Part model, mm, in its own coordinate system. Face numbers are marked on the shaded views. A direction names the side the tool comes from. Round coordinates to 2 decimals unless told otherwise and drop trailing zeros. Loops run counter-clockwise (first coordinate to the right, second up) from the corner with the lowest first, then second, coordinate; pieces in that order, holes last. Notation, with made-up numbers: (80.25, -38.75) -> (118.25, -38.75) arc R16 cw to (118.25, -11.75) -> close; hole circle Ø3 at (49.25, 76.5). An arc over 180 degrees is marked (long way). Use a Markdown table: item, result. Add a question column.
Item 1: Which spindle directions (+Z, -Z, +X, -X, +Y, -Y) get a long thin tool onto all of the face, cutting with end or side? Do the marked faces 4, 5, 6 and 7. Say none if no direction does.
Item 2: Cut at D-D, the plane x = 29. List the corners of the cut face in (y, z), plus the area to 3 significant figures.
Item 3: Flat gauge pins, fed straight in: pin 1 (8 mm diameter, centred on x = -211.5, z = -63, fed in from +Y); pin 2 (4 mm diameter, centred on y = 226, z = -13, fed in from -X); pin 3 (12 mm diameter, centred on x = -229.5, y = 222, fed in from +Z). Where does each tip first touch, or does it go through?
Item 4: Cut at B-B, the plane y = 34.5. List the corners of the cut face in (x, z), plus the area to 3 significant figures.
Item 5: Probe line 1 (X direction, y = 229, z = -59); line 2 (X direction, y = 29, z = -60); line 3 (Z direction, x = 96, y = 67). List the from-to ranges inside material, lowest first. Write a range as [from, to].
Item 6: Cut at A-A, the plane x = -135. List the corners of the cut face in (y, z).
Item 7: Cut at C-C, the plane z = 90. List the corners of the cut face in (x, y).
Item 8: Two-plate mould, pull along X, no slides. Class the marked faces 1, 2 and 3: pulls with the +X half, pulls with the -X half, needs draft (parallel to the pull), parting line crosses it, or undercut.
```python
from build123d import *

# Parameters (mm, degrees)
SKETCH1_W                = 400
SKETCH1_H                = 300
BOSS_EXTRUDE1_DEPTH      = 85
SKETCH2_R                = 65
BOSS_EXTRUDE2_DEPTH      = 200
FILLET1_R                = 30
CUT_EXTRUDE1_DEPTH       = 30
RIB1_REACH               = 408.602
SKETCH4_WALL_W           = 996.380250876
SKETCH4_WALL_H           = 30
SKETCH6_R                = 30
CUT_EXTRUDE2_DEPTH       = 380.110801745
SKETCH7_R                = 45
CUT_EXTRUDE3_DEPTH       = 40
CUT_EXTRUDE4_START       = -40
SKETCH8_R                = 45
CUT_EXTRUDE4_DEPTH       = 40
CHAMFER1_SIZE            = 2
BOSS_EXTRUDE3_REACH      = 547.275
BOSS_EXTRUDE3_END_RADIUS = 65
SKETCH9_W                = 16
SKETCH9_H                = 40
FILLET2_R                = 20
CUT_EXTRUDE5_DEPTH       = 424.826615493
CUT_EXTRUDE5_DEPTH_BACK  = 424.826615493
SKETCH10_R               = 10


with BuildPart() as part:
    # Sketch1 → Boss-Extrude1 (new body)
    with BuildSketch(Plane(origin=(0, 0, 0), x_dir=(1, 0, 0), z_dir=(0, 1, 0))):
        Rectangle(SKETCH1_W, SKETCH1_H)
    extrude(amount=BOSS_EXTRUDE1_DEPTH)

    # Sketch2 → Boss-Extrude2 (add)
    with BuildSketch(Plane(origin=(0, 85, 0), x_dir=(1, 0, 0), z_dir=(0, 1, 0))):
        with Locations(Location((-135, 60, 0), (0, 0, 180))):
            Circle(SKETCH2_R)
    extrude(amount=BOSS_EXTRUDE2_DEPTH)

    # Fillet1
    fillet1_edges = [part.edges().sort_by_distance(p)[0] for p in [
        (200, 42.5, 150),
        (-200, 42.5, 150),
        (-200, 42.5, -150),
        (200, 42.5, -150),
    ]]
    fillet(fillet1_edges, radius=FILLET1_R)

    # Sketch3 → Cut-Extrude1 (cut)
    with BuildSketch(Plane(origin=(0, 85, 0), x_dir=(1, 0, 0), z_dir=(0, 1, 0))):
        with BuildLine():
            Line((70, -70), (170, -70))
            ThreePointArc((170, -70), (190, -90), (170, -110))
            Line((170, -110), (70, -110))
            ThreePointArc((70, -110), (50, -90), (70, -70))
        make_face()
    extrude(amount=-CUT_EXTRUDE1_DEPTH, mode=Mode.SUBTRACT)

    # Sketch4 wall → Rib1 (add, up to next)
    with BuildSketch(Plane(origin=(-27.5, 165, -60), x_dir=(-0.469155225962, 0.883115719457, 0), z_dir=(-0.883115719457, -0.469155225962, 0)), mode=Mode.PRIVATE) as rib1_sk1:
        Rectangle(SKETCH4_WALL_W, SKETCH4_WALL_H)
    rib1_tool1 = extrude(rib1_sk1.sketch, amount=RIB1_REACH, mode=Mode.PRIVATE) - part.part
    add(rib1_tool1.solids().sort_by_distance((-27.5, 165, -60))[0])

    # Sketch6 → Cut-Extrude2 (cut, through all)
    with BuildSketch(Plane(origin=(0, 285, 0), x_dir=(1, 0, 0), z_dir=(0, 1, 0))):
        with Locations(Location((-135, 60, 0), (0, 0, 270))):
            Circle(SKETCH6_R)
    extrude(amount=-CUT_EXTRUDE2_DEPTH, mode=Mode.SUBTRACT)

    # Sketch7 → Cut-Extrude3 (cut)
    with BuildSketch(Plane(origin=(0, 0, 0), x_dir=(1, 0, 0), z_dir=(0, 1, 0))):
        with Locations(Location((-135, 60, 0), (0, 0, 270))):
            Circle(SKETCH7_R)
    extrude(amount=CUT_EXTRUDE3_DEPTH, mode=Mode.SUBTRACT)

    # Sketch8 → Cut-Extrude4 (cut)
    with BuildSketch(Plane(origin=(0, 285, 0), x_dir=(1, 0, 0), z_dir=(0, 1, 0)).offset(CUT_EXTRUDE4_START)):
        with Locations(Location((-135, 60, 0), (0, 0, 270))):
            Circle(SKETCH8_R)
    extrude(amount=CUT_EXTRUDE4_DEPTH, mode=Mode.SUBTRACT)

    # Chamfer1
    chamfer1_edges = [part.edges().sort_by_distance(p)[0] for p in [
        (-135, 285, -105),
        (-135, 245, -90),
        (-135, 40, -90),
        (-135, 0, -105),
    ]]
    chamfer(chamfer1_edges, length=CHAMFER1_SIZE)

    # Boss-Extrude3: up to this cylinder (the profile starts outside it)
    boss_extrude3_end = Plane(origin=(-135, 229, -60), z_dir=(0, -1, 0)) * Cylinder(BOSS_EXTRUDE3_END_RADIUS, 1225.55, mode=Mode.PRIVATE)
    # Sketch9 → Boss-Extrude3 (add, up to the surface)
    with BuildSketch(Plane.ZY.offset(240), mode=Mode.PRIVATE) as boss_extrude3_sk1:
        with Locations((-60, 229)):
            Rectangle(SKETCH9_W, SKETCH9_H)
    boss_extrude3_tool1 = extrude(boss_extrude3_sk1.sketch, amount=-BOSS_EXTRUDE3_REACH, mode=Mode.PRIVATE) - boss_extrude3_end
    add(boss_extrude3_tool1.solids().sort_by_distance((-240, 229, -60))[0])

    # Fillet2
    fillet2_edges = [part.edges().sort_by_distance(p)[0] for p in [
        (-240, 209, -60),
        (-240, 249, -60),
    ]]
    fillet(fillet2_edges, radius=FILLET2_R - 0.0001)  # a hair under: the kernel refuses the full size

    # Sketch10 → Cut-Extrude5 (cut, two sides: drawn at the far end of the back side and taken through both)
    with BuildSketch(Plane.XY.offset(-52).offset(-CUT_EXTRUDE5_DEPTH_BACK)):
        with Locations(Location((-220, 229, 0), (0, 0, 270))):
            Circle(SKETCH10_R)
    extrude(amount=CUT_EXTRUDE5_DEPTH + CUT_EXTRUDE5_DEPTH_BACK, mode=Mode.SUBTRACT)


solid = part.part
```
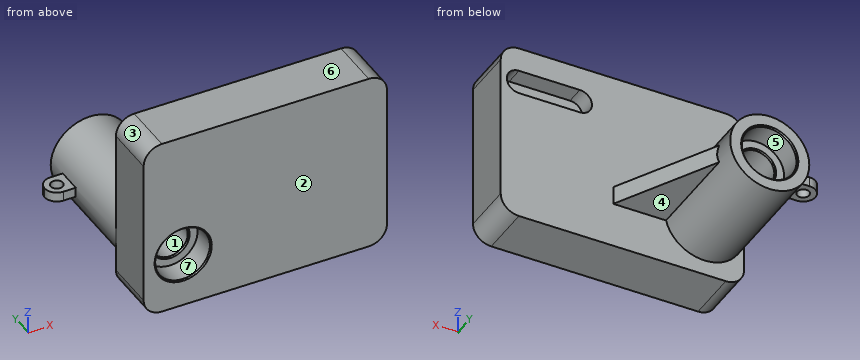
A:
| question | item | result |
|---|---|---|
| 1 | face 4 | -Z, +X, +Y |
| 1 | face 5 | +Y |
| 1 | face 6 | +Z, +X, -X, +Y, -Y |
| 1 | face 7 | -Y |
| 2 | outline | (0, -150) -> (85, -150) -> (85, 150) -> (0, 150) -> close |
| 2 | area | 25,500 mm^2 |
| 3 | pin 1 | stops at y = 249 |
| 3 | pin 2 | stops at x = -181.9 |
| 3 | pin 3 | stops at z = -52 |
| 4 | outline | (-200, -120) arc R30 ccw to (-170, -150) -> (170, -150) arc R30 ccw to (200, -120) -> (200, 120) arc R30 ccw to (170, 150) -> (-170, 150) arc R30 ccw to (-200, 120) -> close; hole circle Ø90 at (-135, -60) |
| 4 | area | 113,000 mm^2 |
| 5 | line 1 | x = [-240, -230], [-210, -164.98], [-105.02, -61.5] |
| 5 | line 2 | x = [-200, -180], [-90, 200] |
| 5 | line 3 | z = [-150, 70], [110, 150] |
| 6 | outline | (0, -150) -> (85, -150) -> (85, -125) -> (285, -125) -> (285, -107) -> (283, -105) -> (245, -105) -> (245, -92) -> (243, -90) -> (42, -90) -> (40, -92) -> (40, -105) -> (2, -105) -> (0, -107) -> close; (0, -13) -> (2, -15) -> (40, -15) -> (40, -28) -> (42, -30) -> (243, -30) -> (245, -28) -> (245, -15) -> (283, -15) -> (285, -13) -> (285, 5) -> (85, 5) -> (85, 150) -> (0, 150) -> close |
| 7 | outline | (-200, 0) -> (200, 0) -> (200, 85) -> (190, 85) -> (190, 55) -> (50, 55) -> (50, 85) -> (-200, 85) -> close |
| 8 | face 1 | undercut |
| 8 | face 2 | needs draft |
| 8 | face 3 | pulls with the -X half |
